```python
from build123d import *

# Parameters (mm, degrees)
F1_DEPTH = 6.35
F2_R     = 0.635


with BuildPart() as f1:
    # F0 (on Top) → F1 (new body)
    with BuildSketch(Plane.XY):
        with BuildLine():
            add(Edge.make_bspline(
                [(-38.9891895168, -10.6982229425), (-38.3465920283, -10.3074894534), (-37.8422569059, -9.6253746617), (-35.8621994283, -5.3779231667), (-35.1209965892, -2.4292102932), (-34.8568920019, -1.175043316)],
                knots=[0, 0, 0, 0, 0.2324380402, 0.6162190201, 1, 1, 1, 1], degree=3))
            Line((-38.9891895168, -10.6982229425), (37.2108104832, -10.6982229425))
            Line((37.2108104832, -10.6982229425), (37.2108104832, 10.6646132435))
            Line((37.2108104832, 10.6646132435), (-34.7275388503, 10.6646132435))
            add(Edge.make_bspline(
                [(-34.7275388503, 10.6646132435), (-34.6275926151, 10.4093259266), (-34.4118404297, 9.6572574945), (-34.3207970154, 6.7101610318), (-34.149913299, 3.9386656499), (-34.416114208, 1.6737423804)],
                knots=[0, 0, 0, 0, 0.1984555205, 0.5308860218, 1, 1, 1, 1], degree=3))
            Line((-34.416114208, 1.6737423804), (-37.0515519649, 2.308008018))
            Line((-37.0515519649, 2.308008018), (-37.0515519649, -1.7913987552))
            Line((-37.0515519649, -1.7913987552), (-34.8568920019, -1.175043316))
        make_face()
        with BuildLine():
            Line((0.7745096379, -1.6043048495), (-10.9163193113, -1.6043048495))
            ThreePointArc((-10.9163193113, -1.6043048495), (-12.5038193113, -0.0168048495), (-10.9163193113, 1.5706951505))
            Line((-10.9163193113, 1.5706951505), (0.7745096379, 1.5706951505))
            ThreePointArc((0.7745096379, 1.5706951505), (2.3620096379, -0.0168048495), (0.7745096379, -1.6043048495))
        make_face(mode=Mode.SUBTRACT)
        with BuildLine():
            Line((29.2821446352, -1.6043048495), (17.9468611174, -1.6043048495))
            ThreePointArc((17.9468611174, -1.6043048495), (16.3593611174, -0.0168048495), (17.9468611174, 1.5706951505))
            Line((17.9468611174, 1.5706951505), (29.2821446352, 1.5706951505))
            ThreePointArc((29.2821446352, 1.5706951505), (30.8696446352, -0.0168048495), (29.2821446352, -1.6043048495))
        make_face(mode=Mode.SUBTRACT)
    extrude(amount=F1_DEPTH)

    # F2
    f2_edges = [f1.edges().sort_by_distance(p)[0] for p in [
        (37.21081, -10.698223, 3.175),
        (-38.98919, -10.698223, 3.175),
        (-0.88919, -10.698223, 0),
        (-0.88919, -10.698223, 6.35),
        (37.21081, -0.016805, 0),
        (37.21081, 10.664613, 3.175),
        (37.21081, -0.016805, 6.35),
        (1.241636, 10.664613, 6.35),
        (1.241636, 10.664613, 0),
        (-10.916319, 1.570695, 3.175),
        (0.77451, 1.570695, 3.175),
        (-5.070905, 1.570695, 0),
        (-5.070905, 1.570695, 6.35),
        (17.946861, 1.570695, 3.175),
        (29.282145, 1.570695, 3.175),
        (23.614503, 1.570695, 0),
        (23.614503, 1.570695, 6.35),
    ]]
    fillet(f2_edges, radius=F2_R)


solid = f1.part
```
Here's how the part is built. I have some questions about the finished solid (model axes, mm). A direction names the side the tool comes from. Coordinates: 2 decimals unless noted, no trailing zeros. Order: outer loops, then holes, each group sorted by start corner. A loop starts at its lowest first (then second) coordinate and runs counter-clockwise, first axis right, second up. Notation, with made-up numbers: (18, -1.75) - (32, -1.75) arc R33 ccw to (32, 33.25) - close; hole circle Ø5 at (-15, 20.25). An arc over 180 degrees is marked (long way). One line per question, with ' | ' between items.
(1) Suppose I cut it at A-A on x = -0.5. List the corners of the cut face in (y, z) for me (3 decimals).
Report:
outline: (-10.698, 0.635) arc R0.635 ccw to (-10.063, 0) - (-2.239, 0) arc R0.635 ccw to (-1.604, 0.635) - (-1.604, 5.715) arc R0.635 ccw to (-2.239, 6.35) - (-10.063, 6.35) arc R0.635 ccw to (-10.698, 5.715) - close; (1.571, 0.635) arc R0.635 ccw to (2.206, 0) - (10.03, 0) arc R0.635 ccw to (10.665, 0.635) - (10.665, 5.715) arc R0.635 ccw to (10.03, 6.35) - (2.206, 6.35) arc R0.635 ccw to (1.571, 5.715) - close
(2) Suppose I cut it at B-B on z = 2. State how many separate pieces and enclosed holes the cut face has, and give its area (3 significant figures).
Report:
separate pieces: 1 | enclosed holes: 2 | area: 1,470 mm2
(3) If we mould it in two halves opening along Y, with no side actions, what happens to faces 4 (the cylindrical face through (-12.5, -0.1, 3.1)), 5 (the flat face through (-0.2, 2.4, 0)), 6 (the flat face through (-1, -10.698, 3)), 7 (the flat face through (-35.97, -1.488, 3.131))? For each: pulls with the +Y half, pulls with the -Y half, needs draft (parallel to the pull), parting line crosses it, or undercut.
Report:
face 4: undercut | face 5: needs draft | face 6: pulls with the -Y half | face 7: undercut
(4) Will this pin go through, and if not, where does the flat tip stop? pin 1 (2 mm diameter, centred on y = -5, z = 5, fed in from -X).
Report:
pin 1: stops at x = -36.26
(5) For faces 1 (the flat face through (-37.052, 0, 3)), 2 (the cylindrical face through (16.36, -0.05, 3.14)), 3 (the flat face through (37.211, 0, 3)), which set-ups out of +Z, -Z, +X, -X, +Y, -Y let a thin tool reach every point of the face, with its end or its side?
Report:
face 1: +Z, -Z, -X, +Y | face 2: +Z, -Z | face 3: +Z, -Z, +X, +Y, -Y
(6) If I drill on L1, parallel to X at y = 0, z = 3; L2, parallel to Y at x = -5.5, z = 2; L3, parallel to X at y = 5.25, z = 3.5, over which ranges is the centre line in solid material (lowest first)?
Report:
L1: x = -37.05 to -12.5, 2.36 to 16.36, 30.87 to 37.21 | L2: y = -10.7 to -1.6, 1.57 to 10.66 | L3: x = -34.25 to 37.21
